Read the model definition and answer for the solid it produces. Units are mm, in the model's axes. Coordinates: 2 decimals unless noted, no trailing zeros. Loops run counter-clockwise (first coordinate to the right, second up) from the corner with the lowest first, then second, coordinate; pieces in that order, holes last.
Q1. Section B-B (y = -0.4) is taken. Give the vertices of the cut face in (x, z).
Q2. Section A-A (z = 0) is taken. Give the vertices of the cut face in (x, y).
Q3. Straight lines are drawn through the part: line 1 (X direction, y = -1.4, z = 12.5); line 2 (Z direction, x = -14, y = -0.8). For each, find the intervals that lie inside material, in ascending order.
Q4. The mould has two halves that part along Z. Classify faces 1 (the face through (-10.84, -0.04, -14.02)), 2 (the face through (-16.07, 0.04, 16)), 3 (the face through (-10.74, -0.04, -2.38)), 4 (the face through (-8, 3, -8)): pulls with the +Z half, pulls with the -Z half, needs draft (parallel to the pull), parting line crosses it, or undercut.
Q5. A flat-ended cylindrical pin translates along its axis: P1, Ø4, axis at x = 12.5, z = 12.5, coming from the +Y side. Find the tip coordinate at first contact, or state that the pin passes through.
Q6. Section C-C (x = 0) is taken. Give the vertices of the cut face in (y, z), then the cut area to 3 significant figures.
from build123d import *

# Parameters (mm, degrees)
CROQUIS1_W                   = 35
CROQUIS1_H                   = 35
CROQUIS1_R                   = 11
SALIENTE_EXTRUIR1_DEPTH      = 3
TALADRO_DE_MARGEN_PARA_M41_D = 4.5
REDONDEO1_R                  = 5


with BuildPart() as part:
    # Croquis1 → Saliente-Extruir1 (new, symmetric)
    with BuildSketch(Plane(origin=(0, 0, 0), x_dir=(1, 0, 0), z_dir=(0, 1, 0))):
        Rectangle(CROQUIS1_W, CROQUIS1_H)
        with Locations(Location((0, 0, 0), (0, 0, 270))):
            Circle(CROQUIS1_R, mode=Mode.SUBTRACT)
    extrude(amount=SALIENTE_EXTRUIR1_DEPTH, both=True)

    # Taladro de margen para M41 (through all)
    with Locations(Plane(origin=(0, 3, 0), x_dir=(1, 0, 0), z_dir=(0, 1, 0))):
        with Locations((12.5, 12.5), (-12.5, 12.5), (-12.5, -12.5), (12.5, -12.5)):
            Hole(TALADRO_DE_MARGEN_PARA_M41_D / 2)

    # Redondeo1
    redondeo1_edges = [part.edges().sort_by_distance(p)[0] for p in [
        (17.5, 0, 17.5),
        (-17.5, 0, 17.5),
        (-17.5, 0, -17.5),
        (17.5, 0, -17.5),
    ]]
    fillet(redondeo1_edges, radius=REDONDEO1_R)


solid = part.part
Numbers:
1. outline: (-17.5, -12.5) arc R5 ccw to (-12.5, -17.5) - (12.5, -17.5) arc R5 ccw to (17.5, -12.5) - (17.5, 12.5) arc R5 ccw to (12.5, 17.5) - (-12.5, 17.5) arc R5 ccw to (-17.5, 12.5) - close; hole circle Ø4.5 at (-12.5, -12.5); hole circle Ø4.5 at (-12.5, 12.5); hole circle Ø22 at (0, 0); hole circle Ø4.5 at (12.5, -12.5); hole circle Ø4.5 at (12.5, 12.5)
2. outline: (-17.5, -3) - (-11, -3) - (-11, 3) - (-17.5, 3) - close; (11, -3) - (17.5, -3) - (17.5, 3) - (11, 3) - close
3. line 1: x = -17.5 to -14.75, -10.25 to 10.25, 14.75 to 17.5
3. line 2: z = -17.27 to -14.18, -10.82 to 10.82, 14.18 to 17.27
4. face 1: undercut
4. face 2: pulls with the +Z half
4. face 3: undercut
4. face 4: needs draft
5. P1: passes through
6. outline: (-3, -17.5) - (3, -17.5) - (3, -11) - (-3, -11) - close; (-3, 11) - (3, 11) - (3, 17.5) - (-3, 17.5) - close
6. area: 78.0 mm2
